```python
from build123d import *

# Parameters (mm, degrees)
SKETCH_W        = 144.02
SKETCH_H        = 69
PAD_DEPTH       = 2
SKETCH001_R     = 1.5
POCKET_DEPTH    = 5
SKETCH002_W     = 23
SKETCH002_H     = 3
PAD001_DEPTH    = 11
SKETCH003_W     = 40
SKETCH003_H     = 69
PAD002_DEPTH    = 2
SKETCH004_W     = 37.3
SKETCH004_H     = 53
PAD003_DEPTH    = 2
SKETCH005_R     = 1.5
POCKET001_DEPTH = 5
SKETCH006_R     = 7
POCKET002_DEPTH = 5
SKETCH007_R     = 1
POCKET003_DEPTH = 5
SKETCH008_R     = 2.5
SKETCH008_W     = 23.5
SKETCH008_H     = 14.25
POCKET004_DEPTH = 5
SKETCH024_R     = 1
POCKET012_DEPTH = 5
SKETCH025_W     = 7
SKETCH025_H     = 9.2
SKETCH025_W_2   = 6.15
SKETCH025_H_2   = 7.35
PAD012_DEPTH    = 2
SKETCH026_W     = 14
SKETCH026_H     = 13
PAD013_DEPTH    = 6.5
SKETCH027_W     = 13
SKETCH027_H     = 1
POCKET013_DEPTH = 10
SKETCH028_W     = 15
SKETCH028_H     = 7
PAD014_DEPTH    = 1
SKETCH038_W     = 12.2
SKETCH038_H     = 11.8
PAD022_DEPTH    = 7
SKETCH039_R     = 3.5
PAD023_DEPTH    = 7
SKETCH040_R     = 3
PAD024_DEPTH    = 8
SKETCH041_W     = 10
SKETCH041_H     = 10
POCKET016_DEPTH = 7
SKETCH042_R     = 7.5
PAD025_DEPTH    = 5
SKETCH043_W     = 57.2
SKETCH043_H     = 18.5
PAD026_DEPTH    = 17
SKETCH044_W     = 12
SKETCH044_H     = 8.19
PAD027_DEPTH    = 3
SKETCH045_W     = 9.7
SKETCH045_H     = 7.15
PAD028_DEPTH    = 7
SKETCH046_R     = 1.2
PAD029_DEPTH    = 4
SKETCH047_W     = 4.85
SKETCH047_H     = 4.45
PAD030_DEPTH    = 6
SKETCH048_R     = 1.5
PAD031_DEPTH    = 4
SKETCH049_W     = 29
SKETCH049_H     = 55.5
PAD032_DEPTH    = 18
SKETCH050_R     = 2.5
PAD033_DEPTH    = 8
SKETCH051_W     = 100
SKETCH051_H     = 60
PAD034_DEPTH    = 12
SKETCH052_R     = 4.5
PAD035_DEPTH    = 16
FILLET003_R     = 4
SKETCH053_W     = 32
SKETCH053_H     = 18.5
POCKET017_DEPTH = 9
SKETCH062_W     = 16.12
SKETCH062_H     = 8
PAD041_DEPTH    = 7


with BuildPart() as part:
    # Sketch → Pad (new body)
    with BuildSketch(Plane.XY):
        Rectangle(SKETCH_W, SKETCH_H)
    extrude(amount=PAD_DEPTH)

    # Sketch001 (on Face6 of Pad) → Pocket (cut)
    with BuildSketch(Plane.XY.offset(2)):
        with Locations((-69.41, -31.7)):
            Circle(SKETCH001_R)
        with Locations((-34.41, -31.7)):
            Circle(SKETCH001_R)
        with Locations((-69.41, 30.8)):
            Circle(SKETCH001_R)
        with Locations((-34.41, 30.8)):
            Circle(SKETCH001_R)
    extrude(amount=-POCKET_DEPTH, mode=Mode.SUBTRACT)

    # Sketch002 (on Face5 of Pocket) → Pad001 (join)
    with BuildSketch(Plane.XY.offset(2)):
        with Locations((-52.51, -33)):
            Rectangle(SKETCH002_W, SKETCH002_H)
    extrude(amount=PAD001_DEPTH)

    # Sketch003 (on Face15 of Pad001) → Pad002 (join)
    with BuildSketch(Plane.XY.offset(13)):
        with Locations((-52.01, 0)):
            Rectangle(SKETCH003_W, SKETCH003_H)
    extrude(amount=PAD002_DEPTH)

    # Sketch004 (on Face6 of Pad002) → Pad003 (join)
    with BuildSketch(Plane.XY.offset(15)):
        with Locations((-51.86, 0)):
            Rectangle(SKETCH004_W, SKETCH004_H)
    extrude(amount=PAD003_DEPTH)

    # Sketch005 (on Face6 of Pad003) → Pocket001 (cut)
    with BuildSketch(Plane.XY.offset(15)):
        with Locations((-69.41, 30.8)):
            Circle(SKETCH005_R)
        with Locations((-34.41, 30.8)):
            Circle(SKETCH005_R)
        with Locations((-34.41, -31.7)):
            Circle(SKETCH005_R)
        with Locations((-69.41, -31.7)):
            Circle(SKETCH005_R)
    extrude(amount=-POCKET001_DEPTH, mode=Mode.SUBTRACT)

    # Sketch006 (on Face23 of Pocket001) → Pocket002 (cut)
    with BuildSketch(Plane(origin=(0, 0, 0), x_dir=(1, 0, 0), z_dir=(0, 0, -1))):
        with Locations((-52.01, -13.75)):
            Circle(SKETCH006_R)
    extrude(amount=-POCKET002_DEPTH, mode=Mode.SUBTRACT)

    # Sketch007 (on Face20 of Pocket002) → Pocket003 (cut)
    with BuildSketch(Plane.XY.offset(2)):
        with Locations((-59.01, 20.8)):
            Circle(SKETCH007_R)
        with Locations((-44.01, 7.8)):
            Circle(SKETCH007_R)
    extrude(amount=-POCKET003_DEPTH, mode=Mode.SUBTRACT)

    # Sketch008 (on Face23 of Pocket003) → Pocket004 (cut)
    with BuildSketch(Plane(origin=(0, 0, 0), x_dir=(1, 0, 0), z_dir=(0, 0, -1))):
        with Locations((-52.01, 4)):
            Circle(SKETCH008_R)
        with Locations((-52.01, 15.625)):
            Rectangle(SKETCH008_W, SKETCH008_H)
    extrude(amount=-POCKET004_DEPTH, mode=Mode.SUBTRACT)

    # Sketch024 (on Face20 of Pocket004) → Pocket012 (cut)
    with BuildSketch(Plane.XY.offset(2)):
        with Locations((-28.99, -13)):
            Circle(SKETCH024_R)
        with Locations((-22.99, 6)):
            Circle(SKETCH024_R)
        with Locations((32.51, 12)):
            Circle(SKETCH024_R)
        with Locations((50.01, 30)):
            Circle(SKETCH024_R)
        with Locations((48.01, -22)):
            Circle(SKETCH024_R)
        with Locations((68.01, -11)):
            Circle(SKETCH024_R)
        with Locations((69.01, 17)):
            Circle(SKETCH024_R)
    extrude(amount=-POCKET012_DEPTH, mode=Mode.SUBTRACT)

    # Sketch025 (on Face20 of Pocket012) → Pad012 (join, symmetric)
    with BuildSketch(Plane.XY.offset(2)):
        with Locations((69.41, 26.6)):
            Rectangle(SKETCH025_W, SKETCH025_H)
        with Locations((70.58, 8.2)):
            Rectangle(SKETCH025_W_2, SKETCH025_H_2)
    extrude(amount=PAD012_DEPTH, both=True)

    # Sketch026 (on Face20 of Pad012) → Pad013 (join)
    with BuildSketch(Plane.XY.offset(2)):
        with Locations((67.143, -25.26)):
            Rectangle(SKETCH026_W, SKETCH026_H)
    extrude(amount=PAD013_DEPTH)

    # Sketch027 (on Face65 of Pad013) → Pocket013 (cut)
    with BuildSketch(Plane.YZ.offset(74.143)):
        with Locations((-25.26, 2.5)):
            Rectangle(SKETCH027_W, SKETCH027_H)
    extrude(amount=-POCKET013_DEPTH, mode=Mode.SUBTRACT)

    # Sketch028 (on Face67 of Pocket013) → Pad014 (join)
    with BuildSketch(Plane.YZ.offset(74.143)):
        with Locations((-25.26, 5.75)):
            Rectangle(SKETCH028_W, SKETCH028_H)
    extrude(amount=-PAD014_DEPTH)

    # Sketch038 (on Face20 of Pad014) → Pad022 (join)
    with BuildSketch(Plane.XY.offset(2)):
        with Locations((-6.01, 0)):
            Rectangle(SKETCH038_W, SKETCH038_H)
    extrude(amount=PAD022_DEPTH)

    # Sketch039 (on Face73 of Pad022) → Pad023 (join)
    with BuildSketch(Plane.XY.offset(9)):
        with Locations((-6.01, 0)):
            Circle(SKETCH039_R)
    extrude(amount=PAD023_DEPTH)

    # Sketch040 (on Face80 of Pad023) → Pad024 (join)
    with BuildSketch(Plane.XY.offset(16)):
        with Locations((-6.01, 0)):
            Circle(SKETCH040_R)
    extrude(amount=PAD024_DEPTH)

    # Sketch041 (on Face83 of Pad024) → Pocket016 (cut)
    with BuildSketch(Plane.XY.offset(24)):
        with Locations((0.49, 0)):
            Rectangle(SKETCH041_W, SKETCH041_H)
    extrude(amount=-POCKET016_DEPTH, mode=Mode.SUBTRACT)

    # Sketch042 (on Face20 of Pocket016) → Pad025 (join)
    with BuildSketch(Plane.XY.offset(2)):
        with Locations((40.89, 19.6)):
            Circle(SKETCH042_R)
    extrude(amount=PAD025_DEPTH)

    # Sketch043 (on Face20 of Pad025) → Pad026 (join)
    with BuildSketch(Plane.XY.offset(2)):
        with Locations((0.37, 25.25)):
            Rectangle(SKETCH043_W, SKETCH043_H)
    extrude(amount=PAD026_DEPTH)

    # Sketch044 (on Face23 of Pad026) → Pad027 (join)
    with BuildSketch(Plane(origin=(0, 0, 0), x_dir=(1, 0, 0), z_dir=(0, 0, -1))):
        with Locations((16.89, 32.055)):
            Rectangle(SKETCH044_W, SKETCH044_H)
    extrude(amount=-PAD027_DEPTH)

    # Sketch045 (on Face20 of Pad027) → Pad028 (join)
    with BuildSketch(Plane.XY.offset(2)):
        with Locations((-26.56, -30.925)):
            Rectangle(SKETCH045_W, SKETCH045_H)
    extrude(amount=PAD028_DEPTH)

    # Sketch046 (on Face23 of Pad028) → Pad029 (join)
    with BuildSketch(Plane.XZ.offset(34.5)):
        with Locations((-26.56, 6)):
            Circle(SKETCH046_R)
    extrude(amount=PAD029_DEPTH)

    # Sketch047 (on Face20 of Pad029) → Pad030 (join)
    with BuildSketch(Plane.XY.offset(2)):
        with Locations((-16.61, -32.275)):
            Rectangle(SKETCH047_W, SKETCH047_H)
    extrude(amount=PAD030_DEPTH)

    # Sketch048 (on Face23 of Pad030) → Pad031 (join)
    with BuildSketch(Plane.XZ.offset(34.5)):
        with Locations((-16.61, 6)):
            Circle(SKETCH048_R)
    extrude(amount=PAD031_DEPTH)

    # Sketch049 (on Face21 of Pad031) → Pad032 (join)
    with BuildSketch(Plane(origin=(0, 0, 0), x_dir=(1, 0, 0), z_dir=(0, 0, -1))):
        with Locations((-52.01, -2)):
            Rectangle(SKETCH049_W, SKETCH049_H)
    extrude(amount=PAD032_DEPTH)

    # Sketch050 (on Face21 of Pad032) → Pad033 (join)
    with BuildSketch(Plane(origin=(0, 0, 0), x_dir=(1, 0, 0), z_dir=(0, 0, -1))):
        Circle(SKETCH050_R)
    extrude(amount=PAD033_DEPTH)

    # Sketch051 (on Face112 of Pad033) → Pad034 (join)
    with BuildSketch(Plane(origin=(0, 0, -8), x_dir=(1, 0, 0), z_dir=(0, 0, -1))):
        with Locations((18, 0)):
            Rectangle(SKETCH051_W, SKETCH051_H)
    extrude(amount=PAD034_DEPTH)

    # Sketch052 (on Face10 of Pad034) → Pad035 (join)
    with BuildSketch(Plane(origin=(-72.01, 0, 0), x_dir=(0, -1, 0), z_dir=(-1, 0, 0))):
        with Locations((-5.1, 2)):
            Circle(SKETCH052_R)
        with Locations((5.1, 2)):
            Circle(SKETCH052_R)
    extrude(amount=PAD035_DEPTH)

    # Fillet003
    fillet003_edges = [part.edges().sort_by_distance(p)[0] for p in [
        (-88.01, 9.6, 2),
        (-88.01, -0.6, 2),
    ]]
    fillet(fillet003_edges, radius=FILLET003_R)

    # Sketch053 (on Face87 of Fillet003) → Pocket017 (cut)
    with BuildSketch(Plane.XY.offset(11)):
        with Locations((-12.23, 25.25)):
            Rectangle(SKETCH053_W, SKETCH053_H)
    extrude(amount=POCKET017_DEPTH, mode=Mode.SUBTRACT)

    # Sketch062 (on Face9 of Pocket017) → Pad041 (join)
    with BuildSketch(Plane.XY.offset(2)):
        with Locations((-20.17, 12)):
            Rectangle(SKETCH062_W, SKETCH062_H)
    extrude(amount=PAD041_DEPTH)


solid = part.part
```
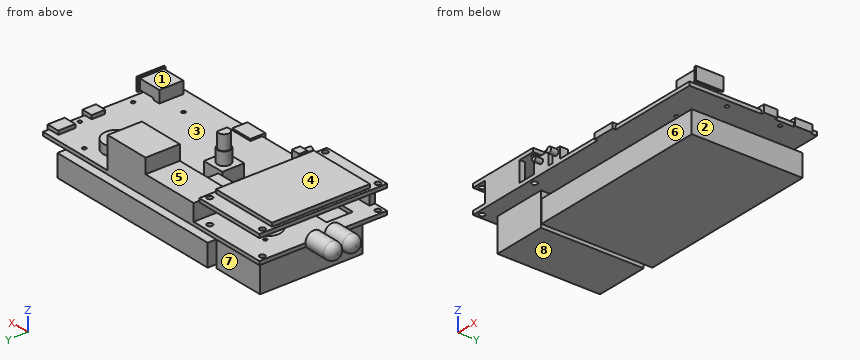
Input: part model. Units: mm. Frame: model coordinates. Face numbers are marked on the shaded views. A direction names the side the tool comes from. Give positions to 0.01 mm unless a question says otherwise; leave off trailing zeros. Write each loop counter-clockwise with the first axis right and the second up, starting at its lowest first coordinate (ties: lowest second). Pieces come first, ordered by that corner, then holes. Notation, with made-up numbers: (-34.75, 56) - (14.25, 56) arc R18 cw to (14.25, 91) - close; hole circle Ø4 at (44.25, -18.5). An arc over 180 degrees is marked (long way). Write item = value, one per line. Start each with the question number.
1) Pin query (flat end, axial travel): pin 1 (2 mm diameter, centred on x = 24, z = -8.5, fed in from +Y); pin 2 (8 mm diameter, centred on x = -25, y = -30.5, fed in from +Z); pin 3 (1.6 mm diameter, centred on x = -59.01, y = 20.8, fed in from +Z); pin 4 (5 mm diameter, centred on x = -33.5, z = -4, fed in from -Y). Return the tip coordinate at first contact, or that it passes through.
2) Cut plane C-C (z = -5.5). Return loops of the section in (x, y).
3) Material intervals for L1, parallel to Z at x = 8, y = -11.5; L2, parallel to Z at x = -53, y = -8; L3, parallel to X at y = -9, z = -17.5, sorted ascending. Write a range as [from, to].
4) Reachability of the marked faces 4, 5, 6, 7 and 8 from +Z, -Z, +X, -X, +Y, -Y: full face, straight path, thin tool, end or side. Return the list, or none.
5) Cut plane A-A (z = -12.5). Return loops of the section in (x, y).
6) Cut plane D-D (x = -73.5). Return loops of the section in (y, z).
7) Draft query along Z for the marked faces 1, 2 and 3. Return one class per face: pulls with the +Z half, pulls with the -Z half, needs draft (parallel to the pull), parting line crosses it, or undercut.
8) Cut plane B-B (x = 12.5). Return loops of the section in (y, z).
Answers follow:
q1.pin_1 = 30
q1.pin_2 = 9
q1.pin_3 = 17
q1.pin_4 = through
q2.outline = (-66.51, -25.75) - (-37.51, -25.75) - (-37.51, 29.75) - (-66.51, 29.75) - close; circle Ø5 at (0, 0)
q3.L1 = [-20, -8], [0, 2]
q3.L2 = [-18, 2], [13, 17]
q3.L3 = [-66.51, -37.51], [-32, 68]
q4.face_4 = +Z, -X, +Y, -Y
q4.face_5 = +Z, -X, +Y
q4.face_6 = -Z, +X, -X, -Y
q4.face_7 = -Z, -X, +Y
q4.face_8 = -Z, -X, +Y, -Y
q5.outline = (-66.51, -25.75) - (-37.51, -25.75) - (-37.51, 29.75) - (-66.51, 29.75) - close; (-32, -30) - (68, -30) - (68, 30) - (-32, 30) - close
q6.outline = circle Ø9 at (-5.1, 2); circle Ø9 at (5.1, 2)
q7.face_1 = pulls with the +Z half
q7.face_2 = needs draft
q7.face_3 = undercut
q8.outline = (-36.15, 0) - (34.5, 0) - (34.5, 19) - (16, 19) - (16, 2) - (-27.96, 2) - (-27.96, 3) - (-36.15, 3) - close; (-30, -20) - (30, -20) - (30, -8) - (-30, -8) - close
